```python
from build123d import *

# Parameters (mm, degrees)
SKETCH1_R      = 3.175
EXTRUDE1_DEPTH = 1.8542
FILLET1_R      = 1.524
SKETCH2_R      = 1.7526
EXTRUDE2_DEPTH = 7.9375
EXTRUDE3_DEPTH = 1.016


with BuildPart() as part:
    # Sketch1 → Extrude1 (new body)
    with BuildSketch(Plane.XY):
        Circle(SKETCH1_R)
    extrude(amount=EXTRUDE1_DEPTH)

    # Fillet1
    fillet1_edges = [part.edges().sort_by_distance(p)[0] for p in [
        (-3.175, 0, 0),
    ]]
    fillet(fillet1_edges, radius=FILLET1_R)

    # Sketch2 → Extrude2 (add)
    with BuildSketch(Plane.XY.offset(1.8542)):
        Circle(SKETCH2_R)
    extrude(amount=EXTRUDE2_DEPTH)

    # Sketch3 → Extrude3 (cut)
    with BuildSketch(Plane(origin=(0, 0, 0), x_dir=(-1, 0, 0), z_dir=(0, 0, -1))):
        Polygon((0.59085384, 0.981566666), (-0.554634748, 1.002477769), (-1.145488588, 0.020911103), (-0.59085384, -0.981566666), (0.554634748, -1.002477769), (1.145488588, -0.020911103), align=None)
    extrude(amount=-EXTRUDE3_DEPTH, mode=Mode.SUBTRACT)


solid = part.part
```
Build history of the part. All positions in model axes, mm. A direction names the side the tool comes from. Round coordinates to 2 decimals unless told otherwise and drop trailing zeros. Order: outer loops, then holes, each group sorted by start corner. A loop starts at its lowest first (then second) coordinate and runs counter-clockwise, first axis right, second up. Notation, with made-up numbers: (52.25, 30.25) -> (106.25, 30.25) arc R6 cw to (106.25, 41.25) -> close; hole circle Ø3 at (41.25, -12.75). An arc over 180 degrees is marked (long way). Answer in a Markdown table with one row per item.
1) Mould opens along Y. For faces 4 (the flat face through (0.846, 0.519, 0.501)), 5 (the cylindrical face through (-0.69, -3.1, 1.69)), 6 (the flat face through (-0.846, -0.519, 0.501)), 7 (the flat face through (0, 0, 9.792)) say: released by +Y, released by -Y, zero draft, split by the parting line, or undercut.
Values:
| item | result |
|---|---|
| face 4 | undercut |
| face 5 | split by the parting line |
| face 6 | undercut |
| face 7 | zero draft |
2) Band-saw the part on C-C on x = 0. Give the cut face in (y, z) (3 decimals), and give its area (3 significant figures).
Values:
| item | result |
|---|---|
| outline | (-3.175, 1.524) arc R1.524 ccw to (-1.651, 0) -> (-0.992, 0) -> (-0.992, 1.016) -> (0.992, 1.016) -> (0.992, 0) -> (1.651, 0) arc R1.524 ccw to (3.175, 1.524) -> (3.175, 1.854) -> (1.753, 1.854) -> (1.753, 9.792) -> (-1.753, 9.792) -> (-1.753, 1.854) -> (-3.175, 1.854) -> close |
| area | 36.6 mm2 |
3) Pin check, flat tips, straight feed: P1, Ø3, axis at x = 0.5, y = -2, coming from the +Z side; P2, Ø1.5, axis at x = -2, z = 6, coming from the -Y side; P3, Ø1.5, axis at x = -1.5, z = 3, coming from the +Y side. Stop position of each tip, or through.
Values:
| item | result |
|---|---|
| P1 | z = 9.79 |
| P2 | y = -1.23 |
| P3 | y = 1.58 |
4) Band-saw the part on A-A on z = 0.75. Give the cut face in (x, y).
Values:
| item | result |
|---|---|
| outline | circle Ø5.93 at (0, 0); hole (-1.15, -0.02) -> (-0.55, -1) -> (0.59, -0.98) -> (1.15, 0.02) -> (0.55, 1) -> (-0.59, 0.98) -> close |
5) Which spindle directions (+Z, -Z, +X, -X, +Y, -Y) get a long thin tool onto all of the face, cutting with end or side? Do faces 1 (the flat face through (-1, -1, 0)), 2 (the flat face through (0.872, -0.473, 0.501)), 3 (the cylindrical face through (1.67, 0.53, 5.77)). Say none if no direction does.
Values:
| item | result |
|---|---|
| face 1 | -Z, +X, -X, +Y, -Y |
| face 2 | -Z |
| face 3 | +Z |
6) Wall check: L1, parallel to Z at x = 0.75, y = -0.5; L2, parallel to Y at x = 0, z = 4; L3, parallel to X at y = -0.5, z = 4. Give the ranges that are in metal, low to high.
Values:
| item | result |
|---|---|
| L1 | 1.02 to 9.79 |
| L2 | -1.75 to 1.75 |
| L3 | -1.68 to 1.68 |
7) Band-saw the part on B-B on z = 7.5. Give the cut face in (x, y).
Values:
| item | result |
|---|---|
| outline | circle Ø3.51 at (0, 0) |
